Autodesk Inventor part; units mm, degrees
ref_plane "YZ Plane" through (0, 0, 0) normal (1, 0, 0) x (0, 1, 0)
ref_plane "XZ Plane" through (0, 0, 0) normal (0, 1, 0) x (-1, 0, 0)
ref_plane "XY Plane" through (0, 0, 0) normal (0, 0, 1) x (1, 0, 0)
sketch "Sketch11" plane through (0, 0, 0) normal (1, 0, 0) x (0, 1, 0)
  line L0 (0, -6.5) -> (0, 6.5)
  line L1 (0, -6.5) -> (14, -6.5)
  line L2 (14, -6.5) -> (14, -2.5)
  line L3 (14, -2.5) -> (10, -2.5)
  line L4 (10, -2.5) -> (10, 6.5)
  line L5 (10, 6.5) -> (0, 6.5)
  point P0 (0, 0)
  point P1 (0, 0)
  dimension "d50" = 20
  dimension "d51" = 28
  dimension "d52" = 4
  dimension "d53" = 13
revolve "Revolution1" add sketch "Sketch11" angle 360 about axis through (0, 0, -6.5) along (0, 0, 1)
sketch "Sketch12" plane through (0, 0, -6.5) normal (0, 0, -1) x (-1, 0, 0)
  circle A0 centre (0, 0) radius 14
  point P0 (0, 0)
hole "Hole4" at (0, 0, -6.5) direction (0, 0, 1) diameter 6.6 end through all counterbore diameter 11 counterbore depth 6.5
chamfer "Chamfer1" distance 0.5 angle 45 3 edges at (0, -10, 6.5) (0, -14, -2.5) (0, -14, -6.5)
properties part number "TL20240701-10110CV-006" material "S45C"
Source: CAD feature listing. Evaluate the final solid. Frame: model axes, mm. A direction names the side the tool comes from. Round coordinates to 2 decimals unless told otherwise and drop trailing zeros. Loops run counter-clockwise (first coordinate to the right, second up) from the corner with the lowest first, then second, coordinate; pieces in that order, holes last.
Q1. Section D-D, the plane z = -5.25. Return loops of the section in (x, y).
Q2. Mould query, pull axis Y, two halves, no side actions, for faces 1 (the face through (5.362, 12.932, -4.479)), 2 (the face through (0, 6, -6.5)), 3 (the face through (0, 4, 0)). Classes: pulls with the +Y half, pulls with the -Y half, needs draft (parallel to the pull), parting line crosses it, or undercut.
Q3. Section C-C, the plane z = 2. Return loops of the section in (x, y).
Q4. Access query for faces 4 (the face through (5.37, -1.19, -3.2)), 5 (the face through (5, -9, -2.5)), 6 (the face through (-2.23, -2.43, 3.3)). Directions: +Z, -Z, +X, -X, +Y, -Y. A direction counts if a zero-diameter tool reaches every point of the face in a straight line with its end or side. Return the directions, or none.
Q5. First-contact query: P1, Ø7.5, axis at x = 0, y = 0, coming from the -Z side; P2, Ø6, axis at x = 2, z = 3, coming from the -Y side. Flat tips, straight axial feed; report the tip coordinate or a pass-through.
Q6. Section A-A, the plane y = 0. Return loops of the section in (x, z).
Q7. Ray query, line 1 (X direction, y = 0, z = 4.5); line 2 (Y direction, x = 0, z = -4.5); line 3 (X direction, y = 0, z = -1.75). Return the intervals inside material, ascending.
Solutions:
1. outline: circle Ø28 at (0, 0); hole circle Ø11 at (0, 0)
2. face 1: parting line crosses it
2. face 2: needs draft
2. face 3: undercut
3. outline: circle Ø20 at (0, 0); hole circle Ø6.6 at (0, 0)
4. face 4: -Z
4. face 5: +Z
4. face 6: +Z, -Z
5. P1: stops at z = 0
5. P2: stops at y = -10
6. outline: (-14, -6) - (-13.5, -6.5) - (-5.5, -6.5) - (-5.5, 0) - (-3.3, 0) - (-3.3, 6.5) - (-9.5, 6.5) - (-10, 6) - (-10, -2.5) - (-13.5, -2.5) - (-14, -3) - close; (3.3, 0) - (5.5, 0) - (5.5, -6.5) - (13.5, -6.5) - (14, -6) - (14, -3) - (13.5, -2.5) - (10, -2.5) - (10, 6) - (9.5, 6.5) - (3.3, 6.5) - close
7. line 1: x = -10 to -3.3, 3.3 to 10
7. line 2: y = -14 to -5.5, 5.5 to 14
7. line 3: x = -10 to -5.5, 5.5 to 10
